Here's how the part is built. I have some questions about the finished solid (model axes, mm). A direction names the side the tool comes from. Round coordinates to 2 decimals unless told otherwise and drop trailing zeros. Loops run counter-clockwise (first coordinate to the right, second up) from the corner with the lowest first, then second, coordinate; pieces in that order, holes last. Notation, with made-up numbers: M -26.5,84 L 27.5,84 A9 cw 27.5,95 Z; hole C -13,83.5 d5. An arc over 180 degrees is marked long. Answer as a JSON object with one key per item and string values.
from build123d import *

# Parameters (mm, degrees)
SKETCH1_W           = 20
SKETCH1_H           = 10
BOSS_EXTRUDE1_DEPTH = 12
SKETCH2_W           = 7.749887486
SKETCH2_H           = 10
CUT_EXTRUDE1_DEPTH  = 8
FILLET1_R           = 4
SKETCH3_R           = 1.75
CUT_EXTRUDE2_DEPTH  = 21
FILLET2_R           = 3
SKETCH4_R           = 1.75
CUT_EXTRUDE3_DEPTH  = 5


with BuildPart() as part:
    # Sketch1 → Boss-Extrude1 (new body)
    with BuildSketch(Plane(origin=(0, 0, 0), x_dir=(1, 0, 0), z_dir=(0, 1, 0))):
        Rectangle(SKETCH1_W, SKETCH1_H)
    extrude(amount=BOSS_EXTRUDE1_DEPTH)

    # Sketch2 → Cut-Extrude1 (cut)
    with BuildSketch(Plane(origin=(0, 12, 0), x_dir=(1, 0, 0), z_dir=(0, 1, 0))):
        Rectangle(SKETCH2_W, SKETCH2_H)
    extrude(amount=-CUT_EXTRUDE1_DEPTH, mode=Mode.SUBTRACT)

    # Fillet1
    fillet1_edges = [part.edges().sort_by_distance(p)[0] for p in [
        (-6.937471871, 12, -5),
        (6.937471871, 12, 5),
        (-6.937471871, 12, 5),
        (6.937471871, 12, -5),
    ]]
    fillet(fillet1_edges, radius=FILLET1_R)

    # Sketch3 → Cut-Extrude2 (cut, through all)
    with BuildSketch(Plane(origin=(10, 0, 0), x_dir=(0, 0, -1), z_dir=(1, 0, 0))):
        with Locations((0, 8)):
            Circle(SKETCH3_R)
    extrude(amount=-CUT_EXTRUDE2_DEPTH, mode=Mode.SUBTRACT)

    # Fillet2
    fillet2_edges = [part.edges().sort_by_distance(p)[0] for p in [
        (-10, 0, 0),
        (10, 0, 0),
    ]]
    fillet(fillet2_edges, radius=FILLET2_R)

    # Sketch4 → Cut-Extrude3 (cut, through all)
    with BuildSketch(Plane(origin=(0, 4, 0), x_dir=(1, 0, 0), z_dir=(0, 1, 0))):
        Circle(SKETCH4_R)
    extrude(amount=-CUT_EXTRUDE3_DEPTH, mode=Mode.SUBTRACT)


solid = part.part
Item 1: I want a section at C-C, the plane x = -4.25. Please give me the cut outline in (y, z).
Resolved:
{"outline": "M 0,-5 L 8,-5 A4 ccw 12,-1 L 12,1 A4 ccw 8,5 L 0,5 Z; hole C 8,0 d3.5"}
Item 2: I want a section at A-A, the plane y = 6. Please give me the cut outline in (x, z).
Resolved:
{"outline": "M -10,-5 L -3.87,-5 L -3.87,5 L -10,5 Z; M 3.87,-5 L 10,-5 L 10,5 L 3.87,5 Z"}
Item 3: I'm going to push flat-ended pins straight in: pin 1 Ø2 at (x, z) = (0, 3) entering from +Y; pin 2 Ø3 at (x, z) = (0, 0) entering from +Y. Where does each tip first touch, or does it pass through?
Resolved:
{"pin 1": "y = 4", "pin 2": "through"}
Item 4: If we mould it in two halves opening along Z, with no side actions, what happens to faces 3 (the face through (6.98, 9.735, 0.228)), 4 (the face through (-2, 4, 0)), 5 (the face through (6.98, 10.797, -3.859)), 6 (the face through (-6.895, 10.797, 3.859))? For each: pulls with the +Z half, pulls with the -Z half, needs draft (parallel to the pull), parting line crosses it, or undercut.
Resolved:
{"face 3": "undercut", "face 4": "needs draft", "face 5": "pulls with the -Z half", "face 6": "pulls with the +Z half"}
Item 5: On a 3-axis mill with a long thin cutter (end or side, diameter ignored), from which of +Z, -Z, +X, -X, +Y, -Y can I reach the whole of each face in a straight line? I mean faces 1 (the face through (3.875, 6, -1)), 2 (the face through (-6.895, 9.735, 0.228)). Say none if no direction works.
Resolved:
{"face 1": "+Z, -Z, +Y", "face 2": "+X, -X"}
Item 6: I want a section at D-D, the plane x = 1. Please give me the cut outline in (y, z).
Resolved:
{"outline": "M 0,-5 L 4,-5 L 4,-1.44 L 0,-1.44 Z; M 0,1.44 L 4,1.44 L 4,5 L 0,5 Z"}
Item 7: I want a section at B-B, the plane z = 0. Please give me the cut outline in (x, y), then the cut area to 3 significant figures.
Resolved:
{"outline": "M -10,3 A3 ccw -7,0 L -1.75,0 L -1.75,4 L -3.87,4 L -3.87,6.25 L -10,6.25 Z; M -10,9.75 L -3.87,9.75 L -3.87,12 L -10,12 Z; M 1.75,0 L 7,0 A3 ccw 10,3 L 10,6.25 L 3.87,6.25 L 3.87,4 L 1.75,4 Z; M 3.87,9.75 L 10,9.75 L 10,12 L 3.87,12 Z", "area": "117 mm²"}
Item 8: Please list where these lines run through material, in increasing order: probe 1 along X at (y, z) = (4.5, 0.5); probe 2 along X at (y, z) = (3, 0); probe 3 along Y at (x, z) = (6, 0). Write a range as from..to.
Resolved:
{"probe 1": "-10..-3.87, 3.87..10", "probe 2": "-10..-1.75, 1.75..10", "probe 3": "0..6.25, 9.75..12"}
